CAD build for the part. Positions are in the model's coordinates, mm. Round coordinates to 2 decimals unless told otherwise and drop trailing zeros. Loops run counter-clockwise (first coordinate to the right, second up) from the corner with the lowest first, then second, coordinate; pieces in that order, holes last. Notation, with made-up numbers: M 81,22.25 L 97,22.25 A18 ccw 97,41.25 Z; hole C 31.5,70 d1. An arc over 180 degrees is marked long. Use a Markdown table: item, result. Add a question column.
(1) Band-saw the part on A-A, the plane z = 0. Write the cut outline in (x, y).
(2) Band-saw the part on D-D, the plane z = 26. Write the cut outline in (x, y), and give its area (3 significant figures).
(3) Two-plate mould, pull along X, no slides. Class faces 1 (the face through (-2.75, -334.82, -12.4)), 2 (the face through (-22.025, -325.577, -99.184)), 3 (the face through (21, -660.4, 1)): released by +X, released by -X, zero draft, split by the parting line, or undercut.
(4) Band-saw the part on B-B, the plane x = 0. Write the cut outline in (y, z), and give its area (3 significant figures).
(5) Wall check: L1, parallel to Z at x = 0, y = -260.5; L2, parallel to Z at x = -4.5, y = -84; L3, parallel to X at y = -233, z = 85.5. Give the ranges that are in metal, low to high.
(6) Band-saw the part on C-C, the plane y = -222.5. Write the cut outline in (x, z).
(7) Flat gauge pins, fed straight in: P1, Ø10, axis at x = -55, y = -233.5, coming from the -Z side; P2, Ø1, axis at y = -273, z = 7.5, coming from the -X side; P3, Ø10, axis at x = -15.5, y = -478, coming from the -Z side. Where does each tip first touch, or does it go through?
from build123d import *

# Parameters (mm, degrees)
F0_R     = 101.6
F1_DEPTH = 762
F2_R     = 12.7
F3_DEPTH = 762.001
F4_DEPTH = 101.6


with BuildPart() as f1:
    # F0 (on Front) → F1 (new body)
    with BuildSketch(Plane.XZ):
        Circle(F0_R)
    extrude(amount=F1_DEPTH)

    # F2 (on face) → F3 (cut, through all)
    with BuildSketch(Plane.XZ.offset(762)):
        Circle(F2_R)
    extrude(amount=-F3_DEPTH, mode=Mode.SUBTRACT)

    # F4 (cut): a face of the model
    f4_faces = [f1.faces().sort_by_distance(p)[0] for p in [
        (-98.7263180413, -762, 0),
    ]]
    extrude(f4_faces, amount=-F4_DEPTH, mode=Mode.SUBTRACT)


solid = f1.part
Return value:
| question | item | result |
|---|---|---|
| 1 | outline | M -101.6,-660.4 L -12.7,-660.4 L -12.7,0 L -101.6,0 Z; M 12.7,-660.4 L 101.6,-660.4 L 101.6,0 L 12.7,0 Z |
| 2 | outline | M -98.22,-660.4 L 98.22,-660.4 L 98.22,0 L -98.22,0 Z |
| 2 | area | 130,000 mm^2 |
| 3 | face 1 | undercut |
| 3 | face 2 | split by the parting line |
| 3 | face 3 | zero draft |
| 4 | outline | M -660.4,-101.6 L 0,-101.6 L 0,-12.7 L -660.4,-12.7 Z; M -660.4,12.7 L 0,12.7 L 0,101.6 L -660.4,101.6 Z |
| 4 | area | 117,000 mm^2 |
| 5 | L1 | -101.6 to -12.7, 12.7 to 101.6 |
| 5 | L2 | -101.5 to -11.88, 11.88 to 101.5 |
| 5 | L3 | -54.88 to 54.88 |
| 6 | outline | C 0,0 d203.2; hole C 0,0 d25.4 |
| 7 | P1 | z = -88.45 |
| 7 | P2 | x = -101.36 |
| 7 | P3 | z = -101.06 |
